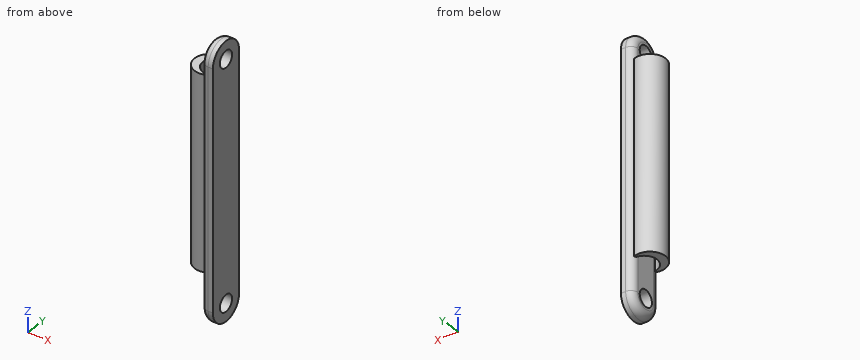
from build123d import *

# Parameters (mm, degrees)
SKETCH002_R                = 3.5
EXTRUDE002_DEPTH           = 5
FILLET002_R                = 3
EXTRUDE025_DEPTH           = 81
EXTRUDE025_ROLL_ANGLE      = -90
EXTRUDE025_PLACEMENT_ANGLE = 180


with BuildPart() as obj1:
    # Sketch002 → Extrude002 (new body)
    with BuildSketch(Plane(origin=(0, 0, 0), x_dir=(0, -1, 0), z_dir=(-1, 0, 0))):
        with BuildLine():
            ThreePointArc((-63.107885, 173.903324), (-70.607885, 181.403324), (-78.107885, 173.903324))
            Line((-78.107885, 173.903324), (-78.107885, 73.903324))
            ThreePointArc((-78.107885, 73.903324), (-70.607885, 66.403324), (-63.107885, 73.903324))
            Line((-63.107885, 173.903324), (-63.107885, 73.903324))
        make_face()
        with Locations((-70.607885, 73.903324)):
            Circle(SKETCH002_R, mode=Mode.SUBTRACT)
        with Locations((-70.607885, 173.903324)):
            Circle(SKETCH002_R, mode=Mode.SUBTRACT)
    extrude(amount=EXTRUDE002_DEPTH)


with BuildPart() as obj1_1:
    # Extrude002 placement: moved
    add(obj1.part.moved(Location((48, 0, 0))))

    # Fillet002
    fillet002_edges = [obj1_1.edges().sort_by_distance(p)[0] for p in [
        (43, 78.107885, 123.903324),
    ]]
    fillet(fillet002_edges, radius=FILLET002_R)


with BuildPart() as fusion029:
    # Sketch026 → Extrude025 (new body)
    with BuildSketch(Plane.XZ):
        with BuildLine():
            ThreePointArc((-3.873562, -5.219724), (6.5, 0), (-3.873562, 5.219724))
            ThreePointArc((-3.873562, -5.219724), (2.950526, 0), (-3.873562, 5.219724))
        make_face()
    extrude(amount=EXTRUDE025_DEPTH)


with BuildPart() as fusion029_1:
    # Extrude025 roll: moved
    add(fusion029.part.rotate(Axis((0, 0, 0), (1, 0, 0)), EXTRUDE025_ROLL_ANGLE))


with BuildPart() as fusion029_2:
    # Extrude025 placement: moved
    add(fusion029_1.part.moved(Location((41.2, 70.65, 88))).rotate(Axis((41.2, 70.65, 88), (0, 0, 1)), EXTRUDE025_PLACEMENT_ANGLE))

    # Fusion029: union obj1
    add(obj1_1.part)


solid = fusion029_2.part
Design review of the part built by this model. Coordinates are the model's own, in mm. Give positions to 0.01 mm unless a question says otherwise; leave off trailing zeros. Write each loop counter-clockwise with the first axis right and the second up, starting at its lowest first coordinate (ties: lowest second). Pieces come first, ordered by that corner, then holes. Notation, with made-up numbers: M 84,-10.75 L 142,-10.75 A27 cw 142,14.25 Z; hole C -11,80.5 d6. An arc over 180 degrees is marked long. Return JSON: item names as keys, results as strings. Group by question number.
Item 1: Take a section at B-B (z = 141.5). Give the boundary of the cut face in (x, y), plus the area to 3 significant figures.
Item 2: Take a section at D-D (y = 71.25). Count the separate pieces of the cut face and the enclosed holes in it, plus the area to 3 significant figures.
Item 3: Take a section at C-C (x = 47). Give the boundary of the cut face in (y, z).
Item 4: Clearance check with flat-ended pins moving along their axes: pin 1 Ø6 at (x, z) = (37, 114) entering from -Y; pin 2 Ø9 at (y, z) = (70.61, 73.9) entering from -X; pin 3 Ø5 at (x, y) = (40, 75) entering from +Z. State where each tip first meets the part, or that it passes through.
Item 5: Wall thickness on line 1 along Z through (x, y) = (47, 70.75); line 2 along X through (y, z) = (71, 125.5); line 3 along Z through (x, y) = (46.25, 73.25): over which ranges is each line inside the solid? List them lowest first.
Item 6: Take a section at A-A (x = 41.5). Give the boundary of the cut face in (y, z), plus the area to 3 significant figures.
Return value:
{
 "1": {"outline": "M 43.44,64.55 A3 ccw 46,63.11 L 48,63.11 L 48,78.11 L 46,78.11 A3 ccw 43.48,76.74 A6.5 ccw long Z; hole M 43,66.11 L 43,75.11 A3 cw 43.15,76.03 A5.41 ccw 43.12,65.27 A3 cw Z", "area": "122 mm2"},
 "2": {"separate pieces": "4", "enclosed holes": "0", "area": "790 mm2"},
 "3": {"outline": "M 63.11,73.9 A7.5 ccw 78.11,73.9 L 78.11,173.9 A7.5 ccw 63.11,173.9 Z; hole C 70.61,73.9 d7; hole C 70.61,173.9 d7"},
 "4": {"pin 1": "stops at y = 64.26", "pin 2": "stops at x = 43", "pin 3": "stops at z = 169"},
 "5": {"line 1": "z = 66.4 to 70.41, 77.4 to 170.41, 177.4 to 181.4", "line 2": "x = 34.71 to 38.26, 43 to 48", "line 3": "z = 66.88 to 71.61, 76.2 to 171.61, 176.2 to 180.92"},
 "6": {"outline": "M 64.16,88 L 65.69,88 L 65.69,169 L 64.16,169 Z; M 75.61,88 L 77.14,88 L 77.14,169 L 75.61,169 Z", "area": "248 mm2"}
}
